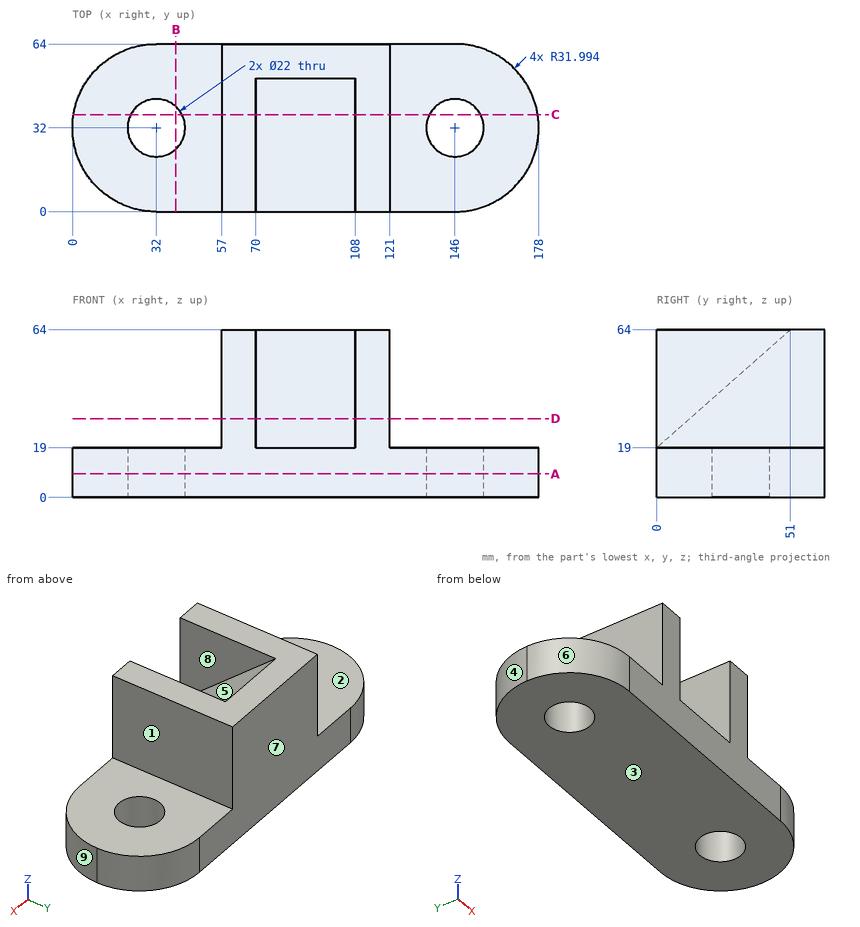
Answer from the drawing. Dimensions are ordinates in mm from the lowest x, y and z of the part. A direction names the side the tool comes from. Round coordinates to 2 decimals unless told otherwise and drop trailing zeros. Order: outer loops, then holes, each group sorted by start corner. A loop starts at its lowest first (then second) coordinate and runs counter-clockwise, first axis right, second up. Notation, with made-up numbers: (79.5, 88) -> (105.5, 88) arc R12 cw to (105.5, 100) -> close; hole circle Ø10 at (-22.75, 57.25). An arc over 180 degrees is marked (long way). Answer as CSV lines item,"result".
Q1. A cutting plane is placed at C-C on y = 37. Determine the outline of the cut face in (x, z), plus the area to 3 significant figures.
Computed values:
outline,"(0.39, 0) -> (22.2, 0) -> (22.2, 19) -> (0.39, 19) -> close; (41.8, 0) -> (136.2, 0) -> (136.2, 19) -> (121, 19) -> (121, 64) -> (108, 64) -> (108, 51.65) -> (70, 51.65) -> (70, 64) -> (57, 64) -> (57, 19) -> (41.8, 19) -> close; (155.8, 0) -> (177.61, 0) -> (177.61, 19) -> (155.8, 19) -> close"
area,"5,030 mm^2"
Q2. A cutting plane is placed at D-D on z = 30. Determine the outline of the cut face in (x, y).
Computed values:
outline,"(57, 0) -> (70, 0) -> (70, 12.47) -> (108, 12.47) -> (108, 0) -> (121, 0) -> (121, 64) -> (57, 64) -> close"
Q3. For a pull along X with two mould halves and no side action, classify the marked faces 6, 7, 8 and 9 as +X half, -X half, draft (parallel to the pull), parting line (faces both ways), or undercut.
Computed values:
face 6,"-X half"
face 7,"draft"
face 8,"undercut"
face 9,"+X half"
Q4. A cutting plane is placed at A-A on z = 9. Give the number of separate pieces and of enclosed holes in the cut face, plus the area to 3 significant figures.
Computed values:
separate pieces,"1"
enclosed holes,"2"
area,"9,750 mm^2"
Q5. A cutting plane is placed at B-B on x = 39.5. Determine the outline of the cut face in (y, z), plus the area to 3 significant figures.
Computed values:
outline,"(0, 0) -> (23.95, 0) -> (23.95, 19) -> (0, 19) -> close; (40.05, 0) -> (64, 0) -> (64, 19) -> (40.05, 19) -> close"
area,"910 mm^2"
Q6. Which of the six approach directions +Z, -Z, +X, -X, +Y, -Y give full straight-line access (tool end or side, diameter ignored) to the marked faces 1, 2, 3, 4 and 5?
Computed values:
face 1,"+Z, +X, +Y, -Y"
face 2,"+Z, -X, +Y, -Y"
face 3,"-Z, +X, -X, +Y, -Y"
face 4,"+Z, -Z, -X, +Y"
face 5,"+Z, -Y"
Q7. Consider line 1 (Y direction, x = 32, z = 5.5); line 2 (X direction, y = 13.5, z = 48); line 3 (X direction, y = 38, z = 17) (1 decimal). Determine where each line is inside the solid, lowest interval first. Write a range as from..to.
Computed values:
line 1,"y = 0..21, 43..64"
line 2,"x = 57..70, 108..121"
line 3,"x = 0.6..22.8, 41.2..136.8, 155.2..177.4"
Q8. Given pin 1 (1 mm diameter, centred on x = 78, z = 52, fed in from -Y) (1 decimal); pin 2 (22.5 mm diameter, centred on y = 40.5, z = 52, fed in from -X); pin 3 (2 mm diameter, centred on x = 43.5, y = 29, fed in from +Z); pin 4 (13 mm diameter, centred on x = 32, y = 32, fed in from +Z), each flat-ended and moving along its own axis, determine where each tip first touches the part or whether it passes through.
Computed values:
pin 1,"stops at y = 36.8"
pin 2,"stops at x = 57"
pin 3,"stops at z = 19"
pin 4,"passes through"
